Part model, mm, in its own coordinate system. Coordinates: 2 decimals unless noted, no trailing zeros. Loops run counter-clockwise (first coordinate to the right, second up) from the corner with the lowest first, then second, coordinate; pieces in that order, holes last. Notation, with made-up numbers: M -16,-19 L 0,-19 A23 ccw 0,8 Z; hole C 6.25,18 d11. An arc over 180 degrees is marked long. Use a Markdown table: item, result. Add a question column.
1) Band-saw the part on C-C (y = -633.5). List the corners of the cut face in (x, z).
2) Band-saw the part on B-B (z = 50.8). List the corners of the cut face in (x, y).
3) Band-saw the part on A-A (x = 25.4). List the corners of the cut face in (y, z).
4) Wall check: probe 1 along X at (y, z) = (-674.5, 50.8); probe 2 along Z at (x, y) = (25, -50); probe 3 along Y at (x, z) = (21.5, 50.8). Give the ranges that are in metal, low to high. Write a range as from..to.
5) Pin check, flat tips, straight feed: pin 1 Ø20.5 at (x, z) = (24.5, 54.5) entering from -Y; pin 2 Ø20.5 at (y, z) = (-355.6, 50.8) entering from +X; pin 3 Ø15 at (x, z) = (25.4, 50.8) entering from -Y; pin 4 Ø7.5 at (x, z) = (28.5, 45.5) entering from +Y. Stop position of each tip, or through.
from build123d import *

# Parameters (mm, degrees)
SKETCH1_W           = 50.8
SKETCH1_H           = 101.6
BOSS_EXTRUDE1_DEPTH = 711.2
SKETCH2_R           = 12.7
CUT_EXTRUDE1_DEPTH  = 50.8
SKETCH3_R           = 12.7
CUT_EXTRUDE2_DEPTH  = 152.4
CUT_EXTRUDE3_START  = -152.4
SKETCH4_R           = 12.7
CUT_EXTRUDE3_DEPTH  = 152.4


with BuildPart() as part:
    # Sketch1 → Boss-Extrude1 (new body)
    with BuildSketch(Plane(origin=(0, 0, 0), x_dir=(1, 0, 0), z_dir=(0, 1, 0))):
        with Locations((25.4, -50.8)):
            Rectangle(SKETCH1_W, SKETCH1_H)
    extrude(amount=-BOSS_EXTRUDE1_DEPTH)

    # Sketch2 → Cut-Extrude1 (cut)
    with BuildSketch(Plane.ZY):
        with Locations((50.8, -355.6)):
            Circle(SKETCH2_R)
    extrude(amount=-CUT_EXTRUDE1_DEPTH, mode=Mode.SUBTRACT)

    # Sketch3 → Cut-Extrude2 (cut)
    with BuildSketch(Plane(origin=(0, 0, 0), x_dir=(1, 0, 0), z_dir=(0, 1, 0))):
        with Locations(Location((25.4, -50.8, 0), (0, 0, 270))):
            Circle(SKETCH3_R)
    extrude(amount=-CUT_EXTRUDE2_DEPTH, mode=Mode.SUBTRACT)

    # Sketch4 → Cut-Extrude3 (cut)
    with BuildSketch(Plane.XZ.offset(711.2).offset(CUT_EXTRUDE3_START)):
        with Locations(Location((25.4, 50.8, 0), (0, 0, 90))):
            Circle(SKETCH4_R)
    extrude(amount=CUT_EXTRUDE3_DEPTH, mode=Mode.SUBTRACT)


solid = part.part
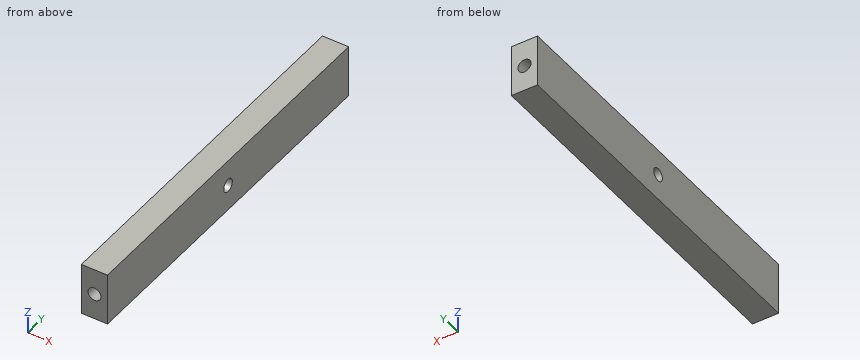
Entries:
| question | item | result |
|---|---|---|
| 1 | outline | M 0,0 L 50.8,0 L 50.8,101.6 L 0,101.6 Z; hole C 25.4,50.8 d25.4 |
| 2 | outline | M 0,-711.2 L 12.7,-711.2 L 12.7,-558.8 L 38.1,-558.8 L 38.1,-711.2 L 50.8,-711.2 L 50.8,-368.3 L 0,-368.3 Z; M 0,-342.9 L 50.8,-342.9 L 50.8,0 L 38.1,0 L 38.1,-152.4 L 12.7,-152.4 L 12.7,0 L 0,0 Z |
| 3 | outline | M -711.2,0 L 0,0 L 0,38.1 L -152.4,38.1 L -152.4,63.5 L 0,63.5 L 0,101.6 L -711.2,101.6 L -711.2,63.5 L -558.8,63.5 L -558.8,38.1 L -711.2,38.1 Z; hole C -355.6,50.8 d25.4 |
| 4 | probe 1 | 0..12.7, 38.1..50.8 |
| 4 | probe 2 | 0..38.11, 63.49..101.6 |
| 4 | probe 3 | -558.8..-368.3, -342.9..-152.4 |
| 5 | pin 1 | y = -711.2 |
| 5 | pin 2 | through |
| 5 | pin 3 | y = -558.8 |
| 5 | pin 4 | y = -152.4 |
